from build123d import *


with BuildPart() as part:
    # Sketch4 → Revolve1 (revolve)
    with BuildSketch(Plane(origin=(0, 0, 0), x_dir=(0, 0, -1), z_dir=(1, 0, 0))):
        with BuildLine():
            Line((-54.61, 0), (0, 0))
            Line((0, 0), (0, 16.51))
            Line((0, 16.51), (-38.1, 16.51))
            ThreePointArc((-38.1, 16.51), (-47.080256121, 20.229743879), (-50.8, 29.21))
            Line((-50.8, 29.21), (-50.8, 379.73))
            ThreePointArc((-50.8, 379.73), (-39.640768363, 406.670768363), (-12.7, 417.83))
            Line((-12.7, 417.83), (0, 417.83))
            Line((0, 417.83), (0, 434.34))
            Line((0, 434.34), (-16.51, 434.34))
            ThreePointArc((-16.51, 434.34), (-52.431024484, 419.461024484), (-67.31, 383.54))
            Line((-67.31, 383.54), (-67.31, 12.7))
            ThreePointArc((-67.31, 12.7), (-63.590256121, 3.719743879), (-54.61, 0))
        make_face()
    revolve(axis=Axis((0, 434.34, 0), (0, -1, 0)))

    # Sketch6 → 3/4 NPT Tapped Hole2 (revolve, cut)
    with BuildSketch(Plane(origin=(0, 434.34, 0), x_dir=(0, 0, 1), z_dir=(1, 0, 0))):
        Polygon((0, 0), (0, 30.027622455), (11.5062, 23.114), (11.5062, 13.97), (12.933217642, 13.97), (13.3324854, 0.635), (13.9674854, 0), align=None)
    revolve(axis=Axis((0, 440.69, 0), (0, -1, 0)), mode=Mode.SUBTRACT)


solid = part.part
Design review of the part built by this model. Coordinates are the model's own, in mm. A direction names the side the tool comes from. Round coordinates to 2 decimals unless told otherwise and drop trailing zeros. Loops run counter-clockwise (first coordinate to the right, second up) from the corner with the lowest first, then second, coordinate; pieces in that order, holes last. Notation, with made-up numbers: (22, -17.75) - (49, -17.75) arc R11 ccw to (49, -2.75) - close; hole circle Ø3 at (45.25, -0.75). An arc over 180 degrees is marked (long way). One line per item, written item: value. Start each with the question number.
1) Consider section A-A on y = 281.5. Give the boundary of the cut face in (x, z).
2) For faces 1 (the flat face through (-1, 0, -1)), 2 (the flat face through (-1, 16.51, 1)), 3 (the cylindrical face through (11.233, 419.118, -2.494)), list the 3-axis set-ups (+Z, -Z, +X, -X, +Y, -Y) from which the entire face can be reached by the end or side of a thin tool; tool diameter is ignored.
3) To check wall thickness, follow L1, parallel to Z at x = 0, y = 295.5; L2, parallel to X at y = 218, z = 2.5. State the ranges of each line that lie inside material, in increasing order. Write a range as from..to.
4) Insertion check: pin 1 Ø4 at (x, z) = (-6, 24) entering from -Y; pin 2 Ø8 at (y, z) = (201, 34) entering from -X; pin 3 Ø3 at (y, z) = (51.5, -45) entering from -X; pin 4 Ø1 at (x, z) = (44.5, -1.5) entering from +Y. Each pin has a flat end and moves straight along its axis. Give the tip position at first contact, or say it passes through.
5) Draft analysis for pull direction X (two halves, no side actions). For faces 4 (the cylindrical face through (65.71, 195.52, -14.59)), 5 (the flat face through (-4, 434.34, 14)), 6 (the cylindrical face through (49.592, 206.924, -11.012)), 7 (the flat face through (-11.3, 417.83, -2.9)), state which applies: +X half, -X half, draft (parallel to the pull), parting line (faces both ways), or undercut.
Reported:
1. outline: circle Ø134.62 at (0, 0); hole circle Ø101.6 at (0, 0)
2. face 1: +Z, -Z, +X, -X, -Y
2. face 2: none
2. face 3: +Y
3. L1: z = -67.31..-50.8, 50.8..67.31
3. L2: x = -67.26..-50.74, 50.74..67.26
4. pin 1: stops at y = 0
4. pin 2: stops at x = -60.25
4. pin 3: stops at x = -51.37
4. pin 4: stops at y = 426.24
5. face 4: parting line
5. face 5: draft
5. face 6: undercut
5. face 7: undercut
